```python
from build123d import *

# Parameters (mm, degrees)
SKETCH2_R                = 10
SKETCH2_R_2              = 7.5
BOSS_EXTRUDE1_DEPTH      = 20
CUT_EXTRUDE1_DEPTH       = 20
SKETCH4_R                = 4.652081996
BOSS_EXTRUDE2_DEPTH      = 50
SKETCH5_R                = 10
SKETCH5_R_2              = 6.506978502
BOSS_EXTRUDE3_DEPTH      = 5
BOSS_EXTRUDE3_DEPTH_BACK = 5


with BuildPart() as part:
    # Sketch2 → Boss-Extrude1 (new body)
    with BuildSketch(Plane.XY):
        Circle(SKETCH2_R)
        Circle(SKETCH2_R_2, mode=Mode.SUBTRACT)
    extrude(amount=BOSS_EXTRUDE1_DEPTH)

    # Sketch3 → Cut-Extrude1 (cut)
    with BuildSketch(Plane.XY.offset(20)):
        with BuildLine():
            Line((-8.852012941, 4.652081996), (-8.852012941, -4.652081996))
            ThreePointArc((-8.852012941, -4.652081996), (-10, 0), (-8.852012941, 4.652081996))
        make_face()
    extrude(amount=-CUT_EXTRUDE1_DEPTH, mode=Mode.SUBTRACT)

    # Sketch4 → Boss-Extrude2 (add)
    with BuildSketch(Plane.ZY.offset(8.852012941)):
        with Locations((10, 0)):
            Circle(SKETCH4_R)
    extrude(amount=BOSS_EXTRUDE2_DEPTH)

    # Sketch5 → Boss-Extrude3 (add, two sides)
    with BuildSketch(Plane(origin=(0, 0, 0), x_dir=(1, 0, 0), z_dir=(0, 1, 0))) as boss_extrude3_sk:
        with Locations((-65.358991443, -10)):
            Circle(SKETCH5_R)
        with Locations((-65.358991443, -10)):
            Circle(SKETCH5_R_2, mode=Mode.SUBTRACT)
    extrude(amount=BOSS_EXTRUDE3_DEPTH)
    extrude(boss_extrude3_sk.sketch, amount=-BOSS_EXTRUDE3_DEPTH_BACK)


solid = part.part
```
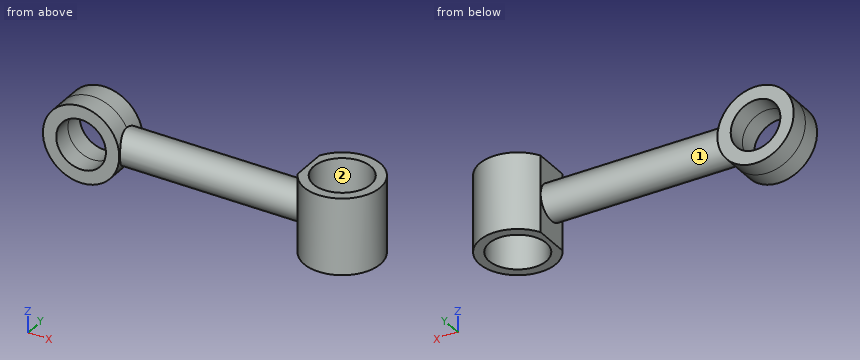
For this review, take the finished solid that the model builds, in its own axes (mm). Face numbers are marked on the shaded views. A direction names the side the tool comes from. Give positions to 0.01 mm unless a question says otherwise; leave off trailing zeros. Loops run counter-clockwise (first coordinate to the right, second up) from the corner with the lowest first, then second, coordinate; pieces in that order, holes last. Notation, with made-up numbers: M 70.25,32.25 L 98.25,32.25 A30 cw 98.25,66.25 Z; hole C -28.5,-11 d8. An arc over 180 degrees is marked long. One line per item, written item: value. Start each with the question number.
Q1. Add section B-B (x = 0). Give the boundary of the cut face in (y, z), and give its area (3 significant figures).
Q2. Add section D-D (x = -28). Give the boundary of the cut face in (y, z), and give its area (3 significant figures).
Q3. Add section A-A (z = 11.25). Give the boundary of the cut face in (x, y), and give its area (3 significant figures).
Q4. Machinability: for the marked faces 1 and 2, which of the approach directions +Z, -Z, +X, -X, +Y, -Y give a long, thin tool a straight path to every point of the face, cutting with its end or side? Answer none if there is none.
Q5. Clearance check with flat-ended pins moving along their axes: pin 1 Ø1 at (x, y) = (-1.5, 7.5) entering from -Z; pin 2 Ø8 at (x, y) = (-16.5, -7.5) entering from +Z; pin 3 Ø6 at (x, z) = (-44, 12) entering from -Y; pin 4 Ø1 at (x, y) = (-53.5, 1.5) entering from +Z. State where each tip first meets the part, or that it passes through.
Q6. For L1, parallel to Y at x = 0, z = 8.25; L2, parallel to X at y = 4.75, z = 18.5; L3, parallel to X at y = -1.6, z = 10, list the stretches that pass through material, from the lowest coordinate up.
Q7. Add section C-C (z = 18.75). Give the boundary of the cut face in (x, y), and give its area (3 significant figures).
Reply:
1. outline: M -10,0 L -7.5,0 L -7.5,20 L -10,20 Z; M 7.5,0 L 10,0 L 10,20 L 7.5,20 Z
1. area: 100 mm²
2. outline: C 0,10 d9.3
2. area: 68.0 mm²
3. outline: M -75.28,-5 L -71.74,-5 L -71.74,5 L -75.28,5 Z; M -58.97,-5 L -55.44,-5 L -55.44,-4.48 L -8.85,-4.48 L -8.85,-4.65 A10 ccw long -8.85,4.65 L -8.85,4.48 L -55.44,4.48 L -55.44,5 L -58.97,5 Z; hole C 0,0 d15
3. area: 618 mm²
4. face 1: none
4. face 2: +Z, -Z
5. pin 1: z = 0
5. pin 2: z = 13.06
5. pin 3: y = -4.65
5. pin 4: z = 14.54
6. L1: -10 to -7.5, 7.5 to 10
6. L2: -70.63 to -60.09, -8.8 to -5.8, 5.8 to 8.8
6. L3: -75.36 to -71.87, -58.85 to -7.33, 7.33 to 9.87
7. outline: M -70.2,-5 L -60.52,-5 L -60.52,5 L -70.2,5 Z; M -8.85,-4.65 A10 ccw long -8.85,4.65 Z; hole C 0,0 d15
7. area: 227 mm²
